Drawing for the job (mm, zero at the part's lowest x, y, z). Round coordinates to 2 decimals unless told otherwise and drop trailing zeros. Write each loop counter-clockwise with the first axis right and the second up, starting at its lowest first coordinate (ties: lowest second). Pieces come first, ordered by that corner, then holes. Notation, with made-up numbers: (53, -24.75) -> (109, -24.75) arc R15 ccw to (109, -7.75) -> close; hole circle Ø8 at (-7.75, -26.5). An arc over 180 degrees is marked (long way). One line per question, with ' | ' between items.
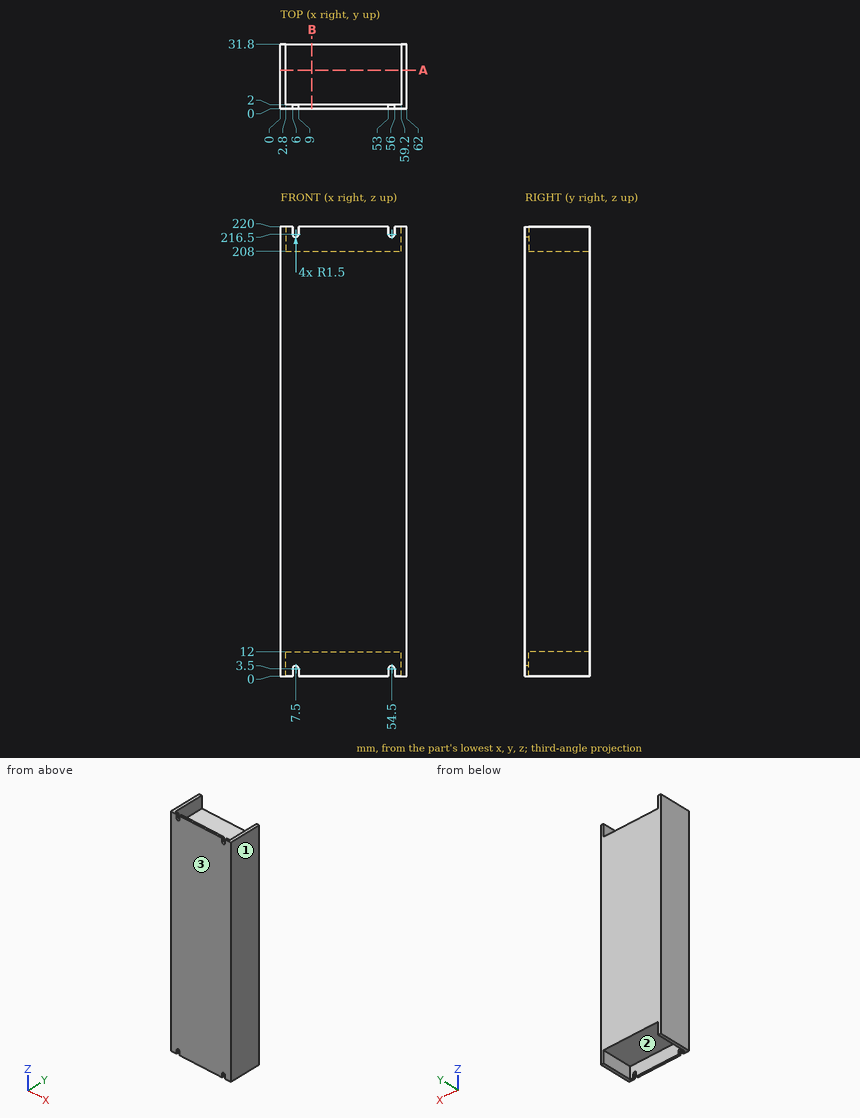
(1) Mould opens along X. For the marked faces 1, 2 and 3 say: pulls with the +X half, pulls with the -X half, needs draft (parallel to the pull), parting line crosses it, or undercut.
Calculated:
face 1: pulls with the +X half | face 2: undercut | face 3: needs draft
(2) Drop flat-ended pins along their axis: pin 1 (1 mm diameter, centred on x = 19, y = 13.5, fed in from -Z); pin 2 (1.5 mm diameter, centred on x = 38.5, z = 100, fed in from -Y); pin 3 (10 mm diameter, centred on x = 32, y = 18.5, fed in from +Z); pin 4 (6 mm diameter, centred on x = 26.5, z = 217, fed in from +Y). Give the stop position or say it passes through.
Calculated:
pin 1: z = 12 | pin 2: y = 0 | pin 3: z = 208 | pin 4: y = 2
(3) Wall check: line 1 (X direction, y = 6.5, z = 210); line 2 (Z direction, x = 54.5, y = 14.5). Give the ranges that are in metal, low to high. Write a range as from..to.
Calculated:
line 1: 0..2.8, 59.2..62 | line 2: 12..208
(4) Slice it at B-B (x = 15.5). Write the cut outline in (y, z), then the cut area to 3 significant figures.
Calculated:
outline: (0, 0) -> (2, 0) -> (2, 12) -> (31.8, 12) -> (31.8, 208) -> (2, 208) -> (2, 220) -> (0, 220) -> close | area: 6,280 mm2
(5) Slice it at A-A (y = 19). Write the cut outline in (x, z), then the cut area to 3 significant figures.
Calculated:
outline: (0, 0) -> (2.8, 0) -> (2.8, 12) -> (59.2, 12) -> (59.2, 0) -> (62, 0) -> (62, 220) -> (59.2, 220) -> (59.2, 208) -> (2.8, 208) -> (2.8, 220) -> (0, 220) -> close | area: 12,300 mm2
